from build123d import *


with BuildPart() as part:
    # Sketch2 → Revolve1 (revolve)
    with BuildSketch(Plane.XY):
        with BuildLine():
            Line((0, 0), (0, 2))
            Line((0, 2), (8, 2))
            Line((8, 2), (8, 3))
            Line((8, 3), (11, 3))
            Line((11, 3), (11, 5))
            Line((11, 5), (14.75, 5.328082488))
            add(Edge.make_bspline(
                [(14.75, 5.328082488), (16.478433804, 2.101172747), (13.75, 0)],
                knots=[0, 0, 0, 1, 1, 1], degree=2))
            Line((13.75, 0), (0, 0))
        make_face()
    revolve(axis=Axis((0, 0, 0), (1, 0, 0)))


solid = part.part
Check sheet for the modelled part. Datum: model origin and axes. Units: mm. A direction names the side the tool comes from. Round coordinates to 2 decimals unless told otherwise and drop trailing zeros. Write each loop counter-clockwise with the first axis right and the second up, starting at its lowest first coordinate (ties: lowest second). Pieces come first, ordered by that corner, then holes. Notation, with made-up numbers: (-20.75, 24.25) - (20.25, 24.25) arc R27 cw to (20.25, 57.25) - close; hole circle Ø6 at (-22.75, -6.5). An arc over 180 degrees is marked (long way). Return JSON: item names as keys, results as strings.
Q1. Scan lines: L1, parallel to X at y = -1.5, z = -2.5; L2, parallel to X at y = 1, z = -4.25; L3, parallel to Z at x = 12, y = 3.5. Record each from-to range of solid material in increasing order. Write a range as from..to.
Returned:
{"L1": "x = 8..15.42", "L2": "x = 11..15.17", "L3": "z = -3.69..3.69"}
Q2. Cross-section at A-A (x = 2.5). Record the boundary of the cut face in (y, z), then the cut area to 3 significant figures.
Returned:
{"outline": "circle Ø4 at (0, 0)", "area": "12.6 mm²"}
Q3. Depth check by flat-ended pin: P1, Ø4, axis at x = 9.5, z = 1, coming from the +Y side; P2, Ø5, axis at x = 5, y = 1.5, coming from the +Z side; P3, Ø5, axis at x = 9.5, y = -3, coming from the -Z side. Enter the tip coordinate at first touch or a pass-through.
Returned:
{"P1": "stops at y = 5.03", "P2": "stops at z = 2", "P3": "stops at z = -4.9"}
Q4. Access from +Z, -Z, +X, -X, +Y, -Y to the whole of each face (thin tool, end or side, straight path). Record for faces 1 (the flat face through (8, -1, -2)), 2 (the flat face through (0, 0, 0)).
Returned:
{"face 1": "-X", "face 2": "+Z, -Z, -X, +Y, -Y"}
Q5. Cross-section at B-B (x = 13.5). Record the boundary of the cut face in (y, z).
Returned:
{"outline": "circle Ø10.44 at (0, 0)"}
